from build123d import *

# Parameters (mm, degrees)
F0_R     = 5
F1_DEPTH = 3
F2_R     = 3
F3_DEPTH = 3
F4_W     = 25
F4_H     = 10
F5_DEPTH = 6
F6_W     = 25
F6_H     = 2.25
F7_DEPTH = 3


with BuildPart() as f1:
    # F0 (on Top) → F1 (new body)
    with BuildSketch(Plane.XY):
        Circle(F0_R)
    extrude(amount=F1_DEPTH)

    # F2 (on Top) → F3 (cut)
    with BuildSketch(Plane.XY):
        Circle(F2_R)
    extrude(amount=F3_DEPTH, mode=Mode.SUBTRACT)

    # F4 (on face) → F5 (join)
    with BuildSketch(Plane.XY.offset(3)):
        Rectangle(F4_W, F4_H)
    extrude(amount=F5_DEPTH)

    # F6 (on face) → F7 (cut)
    with BuildSketch(Plane.XY.offset(9)):
        Rectangle(F6_W, F6_H)
    extrude(amount=-F7_DEPTH, mode=Mode.SUBTRACT)


solid = f1.part
Geometry check sheet. Reference: the model listing, model coordinates, mm. A direction names the side the tool comes from. Coordinates: 2 decimals unless noted, no trailing zeros. Order: outer loops, then holes, each group sorted by start corner. A loop starts at its lowest first (then second) coordinate and runs counter-clockwise, first axis right, second up. Notation, with made-up numbers: M -21,-34.5 L 12,-34.5 A19 cw 12,-20.5 Z; hole C 65,-1.5 d5. An arc over 180 degrees is marked long. Use CSV: the item, a comma, the result in double quotes.
Item 1: Cross-section at A-A on z = 8.25. Record the cut outline in (x, y) (3 decimals).
Returned:
outline,"M -12.5,-5 L 12.5,-5 L 12.5,-1.125 L -12.5,-1.125 Z; M -12.5,1.125 L 12.5,1.125 L 12.5,5 L -12.5,5 Z"
Item 2: Thickness scan on line 1 along Y through (x, z) = (0, 1.4); line 2 along Y through (x, z) = (7.5, 6.75) (3 decimals); line 3 along Z through (x, y) = (2.25, 1.25). Record the ranges inside material, lowest first.
Returned:
line 1,"y = -5 to -3, 3 to 5"
line 2,"y = -5 to -1.125, 1.125 to 5"
line 3,"z = 3 to 9"
Item 3: Cross-section at D-D on z = 2.75. Record the cut outline in (x, y).
Returned:
outline,"C 0,0 d10; hole C 0,0 d6"
Item 4: Cross-section at B-B on y = 0. Record the cut outline in (x, z).
Returned:
outline,"M -12.5,3 L -5,3 L -5,0 L -3,0 L -3,3 L 3,3 L 3,0 L 5,0 L 5,3 L 12.5,3 L 12.5,6 L -12.5,6 Z"
Item 5: Cross-section at C-C on x = 9. Record the cut outline in (y, z) (3 decimals), then the cut area to 4 significant figures.
Returned:
outline,"M -5,3 L 5,3 L 5,9 L 1.125,9 L 1.125,6 L -1.125,6 L -1.125,9 L -5,9 Z"
area,"53.25 mm2"
Item 6: Tool access check on faces 1 (the flat face through (0, 0, 3)), 2 (the flat face through (0, 1.125, 8)), 3 (the flat face through (0, 3, 9)). Record the directions out of +Z, -Z, +X, -X, +Y, -Y that give a thin tool (end or side, any length) a straight path to the whole face; none if there is none.
Returned:
face 1,"-Z"
face 2,"+Z, +X, -X"
face 3,"+Z, +X, -X, +Y, -Y"
Item 7: Mould release check, pull along Y, two halves, no side actions. Record for faces 4 (the flat face through (-12.5, 0, 5)), 5 (the cylindrical face through (-3, 0, 1)), 6 (the flat face through (0, -5, 6)), 7 (the flat face through (0, -1.125, 8)): pulls with the +Y half, pulls with the -Y half, needs draft (parallel to the pull), parting line crosses it, or undercut.
Returned:
face 4,"needs draft"
face 5,"undercut"
face 6,"pulls with the -Y half"
face 7,"undercut"
Item 8: Gauge pin test, flat ends, axial feed: pin 1 Ø0.7 at (x, y) = (1.5, 0.5) entering from +Z; pin 2 Ø1 at (y, z) = (-1.5, 2) entering from +X; pin 3 Ø3 at (x, y) = (7, -1) entering from -Z. Record the tip position at first contact, or that the pin passes through.
Returned:
pin 1,"stops at z = 6"
pin 2,"stops at x = 4.9"
pin 3,"stops at z = 3"
